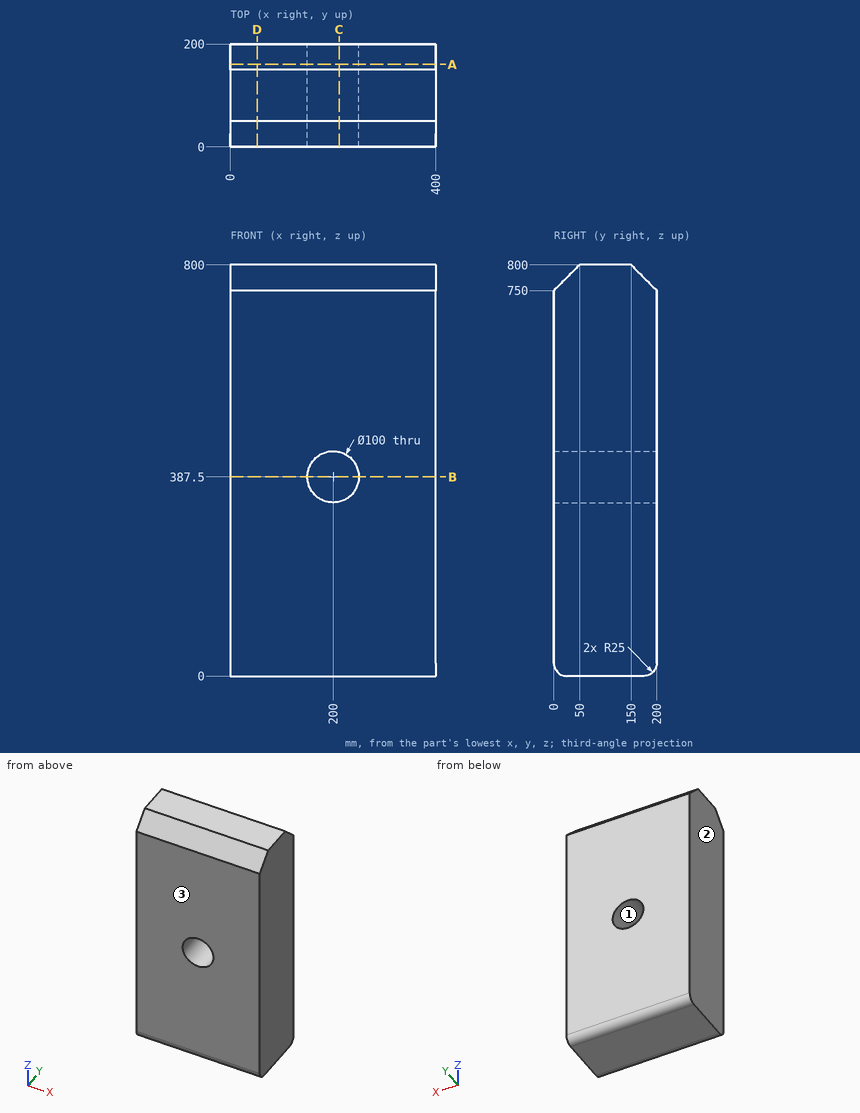
Could you check a few things on this drawing? It's one solid part, dimensions in mm from its lowest x, y, z. Round coordinates to 2 decimals unless told otherwise and drop trailing zeros. Loops run counter-clockwise (first coordinate to the right, second up) from the corner with the lowest first, then second, coordinate; pieces in that order, holes last. Notation, with made-up numbers: M -33.5,4 L 12.5,4 A18 ccw 12.5,38 Z; hole C 87.25,-18.5 d2. An arc over 180 degrees is marked long. Write each question's results on one line, items separated by ' | '. Start each with the question number.
(1) I want a section at C-C (x = 211.5). Please give me the cut outline in (y, z).
(2) I want a section at A-A (y = 160.5). Please give me the cut outline in (x, z), then the cut area to 3 significant figures.
(3) If I drill on probe 1 along Z at (x, y) = (200, 104); probe 2 along Z at (x, y) = (196, 67.5); probe 3 along X at (y, z) = (122, 379.5), over which ranges is the centre line in solid material (lowest first)? Write a range as from..to.
(4) Thinking about a two-plate mould opening in X: for the marked faces 1, 2 and 3, which applies, pulls with the +X half, pulls with the -X half, needs draft (parallel to the pull), parting line crosses it, or undercut?
(5) I want a section at B-B (z = 387.5). Please give me the cut outline in (x, y).
(6) I want a section at D-D (x = 52). Please give me the cut outline in (y, z).
Solved:
1) outline: M 0,25 A25 ccw 25,0 L 175,0 A25 ccw 200,25 L 200,338.84 L 0,338.84 Z; M 0,436.16 L 200,436.16 L 200,750 L 150,800 L 50,800 L 0,750 Z
2) outline: M 0,0 L 400,0 L 400,789.5 L 0,789.5 Z; hole C 200,387.5 d100 | area: 308,000 mm²
3) probe 1: z = 0..337.5, 437.5..800 | probe 2: z = 0..337.66, 437.34..800 | probe 3: x = 0..150.64, 249.36..400
4) face 1: undercut | face 2: pulls with the -X half | face 3: needs draft
5) outline: M 0,0 L 150,0 L 150,200 L 0,200 Z; M 250,0 L 400,0 L 400,200 L 250,200 Z
6) outline: M 0,25 A25 ccw 25,0 L 175,0 A25 ccw 200,25 L 200,750 L 150,800 L 50,800 L 0,750 Z
